from build123d import *

# Parameters (mm, degrees)
CHAMFER1_SIZE      = 1
SKETCH2_R          = 1.5
CUT_EXTRUDE1_DEPTH = 52.176166328
CHAMFER2_SIZE      = 0.5


with BuildPart() as part:
    # Sketch1 → Revolve1 (revolve)
    with BuildSketch(Plane.XY, mode=Mode.PRIVATE) as revolve1_sk:
        Polygon((0, 0), (40, 0), (40, 12.5), (15, 12.5), (15, 25), (3, 25), (3, 6), (0, 6), align=None)
    revolve(revolve1_sk.sketch.rotate(Axis((0, 0, 0), (1, 0, 0)), 90), axis=Axis((0, 0, 0), (1, 0, 0)))

    # Chamfer1
    chamfer1_edges = [part.edges().sort_by_distance(p)[0] for p in [
        (0, 0, -6),
        (3, 0, -25),
    ]]
    chamfer(chamfer1_edges, length=CHAMFER1_SIZE)

    # Sketch2 → Cut-Extrude1 (cut, through all)
    with BuildSketch(Plane.ZY.offset(-3)):
        with Locations((-16, 12)):
            Circle(SKETCH2_R)
        with Locations((0, 20)):
            Circle(SKETCH2_R)
        with Locations((16, 12)):
            Circle(SKETCH2_R)
    extrude(amount=-CUT_EXTRUDE1_DEPTH, mode=Mode.SUBTRACT)

    # Chamfer2
    chamfer2_edges = [part.edges().sort_by_distance(p)[0] for p in [
        (3, 12, -17.5),
        (3, 20, -1.5),
        (3, 12, 14.5),
    ]]
    chamfer(chamfer2_edges, length=CHAMFER2_SIZE)


solid = part.part
Input: part model. Units: mm. Frame: model coordinates. A direction names the side the tool comes from. Coordinates: 2 decimals unless noted, no trailing zeros. Order: outer loops, then holes, each group sorted by start corner. A loop starts at its lowest first (then second) coordinate and runs counter-clockwise, first axis right, second up. Notation, with made-up numbers: M -6,-39 L 37,-39 A23 cw 37,-22 Z; hole C -34,6.5 d7. An arc over 180 degrees is marked long. Write item = value, one per line. Start each with the question number.
(1) Section B-B on x = 8. Output: boundary loops of the cut face in (y, z).
(2) Reachability of faces 4 (the cylindrical face through (9.423, -7.509, 23.846)), 5 (the flat face through (3, -6, 5)), 6 (the cylindrical face through (27.325, -3.755, 11.923)) from +Z, -Z, +X, -X, +Y, -Y: full face, straight path, thin tool, end or side. Return the list, or none.
(3) Section A-A on y = 0. Output: boundary loops of the cut face in (x, z).
(4) First-contact query: P1, Ø4, axis at x = 29, y = -12, coming from the +Z side; P2, Ø2.5, axis at y = 12, z = 16, coming from the -X side; P3, Ø4, axis at y = 8.5, z = -14, coming from the +X side; P4, Ø5, axis at y = 3.5, z = -15, coming from the -X side. Flat tips, straight axial feed; report the tip coordinate or a pass-through.
(5) Section C-C on x = 18. Output: boundary loops of the cut face in (y, z), and give its area (3 significant figures).
(6) Line query: line 1 along Y through (x, z) = (8, 0); line 2 along X through (y, z) = (-11, -1); line 3 along X through (y, z) = (6, 18). Output: solid intervals per line, ascending. Write a range as [from, to].
(7) Pull-direction query (Z, two-part tool) for faces 1 (the flat face through (15, -5.9, 11.5)), 2 (the cylindrical face through (9.17, 12.07, 14.5)), 3 (the cylindrical face through (1.986, -1.802, 5.723)); classes: released by +Z, released by -Z, zero draft, split by the parting line, or undercut.
Result set:
q1.outline = C 0,0 d50; hole C 12,-16 d3; hole C 12,16 d3; hole C 20,0 d3
q2.face_4 = +X, -X
q2.face_5 = -X
q2.face_6 = +X
q3.outline = M 0,-5 L 1,-6 L 3,-6 L 3,-24 L 4,-25 L 15,-25 L 15,-12.5 L 40,-12.5 L 40,12.5 L 15,12.5 L 15,25 L 4,25 L 3,24 L 3,6 L 1,6 L 0,5 Z
q4.P1 = 7.5
q4.P2 = through
q4.P3 = 15
q4.P4 = 3
q5.outline = C 0,0 d25
q5.area = 491 mm²
q6.line_1 = [-25, 18.5], [21.5, 25]
q6.line_2 = [3, 40]
q6.line_3 = [3, 15]
q7.face_1 = zero draft
q7.face_2 = undercut
q7.face_3 = split by the parting line
